Build history of the part. All positions in model axes, mm. A direction names the side the tool comes from. Coordinates: 2 decimals unless noted, no trailing zeros. Loops run counter-clockwise (first coordinate to the right, second up) from the corner with the lowest first, then second, coordinate; pieces in that order, holes last. Notation, with made-up numbers: M 32.5,0.25 L 36.5,0.25 A17 cw 36.5,18.25 Z; hole C 25.25,-18 d10. An arc over 180 degrees is marked long. Write each question's results on one line, items separated by ' | '. Start each with the question number.
from build123d import *

# Parameters (mm, degrees)
SKETCH1_W            = 28.802861634
SKETCH1_H            = 131.078546172
BOSS_EXTRUDE1_DEPTH  = 4
M5_CLEARANCE_HOLE1_D = 5.3
FILLET1_R            = 10
M5_CLEARANCE_HOLE2_D = 5.3
BOSS_EXTRUDE2_DEPTH  = 4
SKETCH8_W            = 47.461989215
SKETCH8_H            = 54.002733852
CUT_EXTRUDE1_DEPTH   = 14.4
FILLET2_R            = 8


with BuildPart() as part:
    # Sketch1 → Boss-Extrude1 (new body)
    with BuildSketch(Plane.XY):
        with Locations((-48.87450938, -319.394379884)):
            Rectangle(SKETCH1_W, SKETCH1_H)
    extrude(amount=BOSS_EXTRUDE1_DEPTH)

    # M5 Clearance Hole1 (through all)
    with Locations(Plane.XY.offset(4)):
        with Locations((-54.16270611, -321.915681156), (-54.16270611, -293.415681156)):
            Hole(M5_CLEARANCE_HOLE1_D / 2)

    # Fillet1
    fillet1_edges = [part.edges().sort_by_distance(p)[0] for p in [
        (-63.275940197, -253.855106798, 2),
        (-34.473078563, -253.855106798, 2),
        (-34.473078563, -384.93365297, 2),
        (-63.275940197, -384.93365297, 2),
    ]]
    fillet(fillet1_edges, radius=FILLET1_R)

    # M5 Clearance Hole2 (through all)
    with Locations(Plane(origin=(0, 0, 0), x_dir=(-1, 0, 0), z_dir=(0, 0, -1))):
        with Locations((45.426427008, -344.165502047)):
            Hole(M5_CLEARANCE_HOLE2_D / 2)

    # Sketch7 → Boss-Extrude2 (add)
    with BuildSketch(Plane.XY.offset(4)):
        Polygon((-63.275940197, -333.655681156), (-105.425150803, -333.655681156), (-105.425150803, -256.153534459), (-79.372706111, -256.153534459), (-79.372706111, -305.639740344), (-63.275940197, -305.639740344), align=None)
    extrude(amount=-BOSS_EXTRUDE2_DEPTH)

    # Sketch8 → Cut-Extrude1 (cut)
    with BuildSketch(Plane(origin=(0, 0, 0), x_dir=(-1, 0, 0), z_dir=(0, 0, -1))):
        with Locations((47.593328547, -278.638373418)):
            Rectangle(SKETCH8_W, SKETCH8_H)
    extrude(amount=-CUT_EXTRUDE1_DEPTH, mode=Mode.SUBTRACT)

    # Fillet2
    fillet2_edges = [part.edges().sort_by_distance(p)[0] for p in [
        (-63.275940197, -333.655681156, 2),
        (-105.425150803, -333.655681156, 2),
        (-105.425150803, -256.153534459, 2),
        (-79.372706111, -256.153534459, 2),
        (-79.372706111, -305.639740344, 2),
        (-34.473078563, -305.639740344, 2),
    ]]
    fillet(fillet2_edges, radius=FILLET2_R)


solid = part.part
1. Mould opens along X. For faces 1 (the cylindrical face through (-53.588, -324.503, 1.972)), 2 (the cylindrical face through (-37.5, -382.1, 2)), 3 (the flat face through (-63.276, -359, 2)) say: +X half, -X half, draft (parallel to the pull), parting line (faces both ways), or undercut.
2. Band-saw the part on C-C, the plane x = -50. List the corners of the cut face in (y, z), plus the area to 3 significant figures.
3. Wall check: line 1 along X through (y, z) = (-371, 2.3); line 2 along X through (y, z) = (-283, 2.15); line 3 along Y through (x, z) = (-80.5, 3.6). Give the ranges that are in metal, low to high.
4. Band-saw the part on B-B, the plane y = -354. List the corners of the cut face in (x, z).
5. Band-saw the part on A-A, the plane z = 1.1. List the corners of the cut face in (x, y).
6. Pin check, flat tips, straight feed: pin 1 (7 mm diameter, centred on x = -54.16, y = -321.92, fed in from -Z); pin 2 (1 mm diameter, centred on x = -70.5, z = 2.5, fed in from -Y); pin 3 (2 mm diameter, centred on x = -50.5, z = 2, fed in from +Y); pin 4 (2 mm diameter, centred on x = -83, z = 2, fed in from +Y). Stop position of each tip, or through.
7. Which spindle directions (+Z, -Z, +X, -X, +Y, -Y) get a long thin tool onto all of the face, cutting with end or side? Do faces 4 (the flat face through (-79.373, -281, 2)), 5 (the flat face through (-84, -333.656, 2)), 6 (the flat face through (-105.425, -295, 2)). Say none if no direction does.
Checked values:
1) face 1: undercut | face 2: +X half | face 3: -X half
2) outline: M -384.93,0 L -305.64,0 L -305.64,4 L -384.93,4 Z | area: 317 mm²
3) line 1: -63.28 to -34.47 | line 2: -105.43 to -79.37 | line 3: -333.66 to -260.06
4) outline: M -63.28,0 L -34.47,0 L -34.47,4 L -63.28,4 Z
5) outline: M -105.43,-325.66 A8 ccw -97.43,-333.66 L -71.28,-333.66 A8 cw -63.28,-341.66 L -63.28,-374.93 A10 ccw -53.28,-384.93 L -44.47,-384.93 A10 ccw -34.47,-374.93 L -34.47,-313.64 A8 ccw -42.47,-305.64 L -71.37,-305.64 A8 cw -79.37,-297.64 L -79.37,-264.15 A8 ccw -87.37,-256.15 L -97.43,-256.15 A8 ccw -105.43,-264.15 Z; hole C -54.16,-321.92 d5.3; hole C -45.43,-344.17 d5.3
6) pin 1: z = 0 | pin 2: y = -333.76 | pin 3: y = -305.64 | pin 4: y = -256.9
7) face 4: +Z, -Z, +X, +Y | face 5: +Z, -Z, -X, -Y | face 6: +Z, -Z, -X, +Y, -Y
